Geometry: final body of the model. Coordinates: model frame, mm. Coordinates: 2 decimals unless noted, no trailing zeros. Loops run counter-clockwise (first coordinate to the right, second up) from the corner with the lowest first, then second, coordinate; pieces in that order, holes last. Notation, with made-up numbers: M 58,29 L 110,29 A28 ccw 110,68 Z; hole C 42,-34 d3. An arc over 180 degrees is marked long. Write each question's results on one line, items separated by ' | '. Start each with the question number.
from build123d import *
from build123d.topology import SkipClean

# Parameters (mm, degrees)
THICKEN1_START     = 3.38125
THICKEN1_DEPTH     = 22.11875
THICKEN1_2_DEPTH   = 1
THICKEN1_START_2   = 1.79375
THICKEN1_3_DEPTH   = 0.79375
THICKEN1_START_3   = 1
THICKEN1_4_DEPTH   = 2.38125
SKETCH7_R          = 0.396875
CUT_EXTRUDE1_DEPTH = 10


with BuildPart() as part:
    # Thicken1: read off the stored shape, not the designer's step
    # Thicken1 outline → Thicken1 (new body)
    with BuildSketch(Plane.XY.offset(THICKEN1_START)):
        with BuildLine():
            ThreePointArc((0, -0.794033341), (0.622, -0.172033341), (0, 0.449966659))
            Line((0, 0.449966659), (0, 0.348580659))
            ThreePointArc((0, 0.348580659), (0.520614, -0.172033341), (0, -0.692647341))
            Line((0, -0.692647341), (0, -0.794033341))
        make_face()
    extrude(amount=THICKEN1_DEPTH)



with BuildPart() as body_2:
    # Thicken1 2 outline → Thicken1 2 (new body)
    with BuildSketch(Plane.XY):
        with BuildLine():
            ThreePointArc((0, -0.794033341), (0.622, -0.172033341), (0, 0.449966659))
            Line((0, 0.449966659), (0, 0.348580659))
            ThreePointArc((0, 0.348580659), (0.520614, -0.172033341), (0, -0.692647341))
            Line((0, -0.692647341), (0, -0.794033341))
        make_face()
    extrude(amount=THICKEN1_2_DEPTH)


with BuildPart() as body_3:
    # Thicken1 3 outline → Thicken1 3 (new body)
    with BuildSketch(Plane.XY.offset(THICKEN1_START_2)):
        with BuildLine():
            ThreePointArc((0, -0.794033341), (0.622, -0.172033341), (0, 0.449966659))
            Line((0, 0.449966659), (0, 0.348580659))
            ThreePointArc((0, 0.348580659), (0.520614, -0.172033341), (0, -0.692647341))
            Line((0, -0.692647341), (0, -0.794033341))
        make_face()
    extrude(amount=THICKEN1_3_DEPTH)


with BuildPart() as part_1:
    add(part.part)

    add(body_2.part)  # Thicken1 4 merges body 2

    add(body_3.part)  # Thicken1 4 merges body 3
    # Thicken1 4 outline → Thicken1 4 (add)
    with BuildSketch(Plane.XY.offset(THICKEN1_START_3)):
        with BuildLine():
            Line((0.40339385, 0.157075059), (0.481952031, 0.221166659))
            ThreePointArc((0.481952031, 0.221166659), (0.26675232, 0.389862735), (0, 0.449966659))
            Line((0, 0.449966659), (0, 0.348580659))
            ThreePointArc((0, 0.348580659), (0.223271692, 0.298273674), (0.40339385, 0.157075059))
        make_face()
    extrude(amount=THICKEN1_4_DEPTH)

    # Sketch7 → Cut-Extrude1 (cut)
    with BuildSketch(Plane(origin=(0, 0, 0), x_dir=(1, 0, 0), z_dir=(0, 1, 0))):
        with Locations((0, -0.5)):
            Circle(SKETCH7_R)
    extrude(amount=-CUT_EXTRUDE1_DEPTH, mode=Mode.SUBTRACT)

    # Mirror2: part across face


with BuildPart() as part_2:
    with SkipClean():  # the faces are left unmerged after this step: merging them gives an invalid solid
        add(part_1.part)
        add(part_1.part.mirror(Plane(origin=(0, 0.399273659, 12.75), x_dir=(0, 0, 1), z_dir=(-1, 0, 0))))


solid = part_2.part
Item 1: Section A-A, the plane x = 0.2. Return loops of the section in (y, z).
Item 2: Section C-C, the plane z = 21. Return loops of the section in (x, y).
Item 3: Section D-D, the plane z = 0.5. Return loops of the section in (x, y), plus the area to 3 significant figures.
Item 4: Ray query, L1, parallel to Z at x = 0.5, y = 0.15; L2, parallel to Y at x = 0.45, z = 11.5. Return the intervals inside material, ascending. Write a range as [from, to].
Item 5: Section B-B, the plane y = -0.1. Return loops of the section in (x, z), plus the area to 3 significant figures.
Solutions:
1) outline: M -0.76,0 L -0.65,0 L -0.65,0.16 L -0.76,0.16 Z; M -0.76,0.84 L -0.65,0.84 L -0.65,1 L -0.76,1 Z; M -0.76,1.79 L -0.65,1.79 L -0.65,2.59 L -0.76,2.59 Z; M -0.76,3.38 L -0.65,3.38 L -0.65,25.5 L -0.76,25.5 Z; M 0.31,0 L 0.42,0 L 0.42,25.5 L 0.31,25.5 Z
2) outline: C 0,-0.17 d1.24; hole C 0,-0.17 d1.04
3) outline: M -0.4,-0.65 L -0.4,-0.51 A0.52 cw long 0.4,-0.51 L 0.4,-0.65 A0.62 ccw long Z | area: 0.275 mm²
4) L1: z = [0, 1], [1.79, 2.59], [3.38, 25.5] | L2: y = [-0.6, -0.43], [0.09, 0.26]
5) outline: M -0.62,0 L -0.52,0 L -0.52,1 L -0.62,1 Z; M -0.62,1.79 L -0.52,1.79 L -0.52,2.59 L -0.62,2.59 Z; M -0.62,3.38 L -0.52,3.38 L -0.52,25.5 L -0.62,25.5 Z; M 0.52,0 L 0.62,0 L 0.62,1 L 0.52,1 Z; M 0.52,1.79 L 0.62,1.79 L 0.62,2.59 L 0.52,2.59 Z; M 0.52,3.38 L 0.62,3.38 L 0.62,25.5 L 0.52,25.5 Z | area: 4.89 mm²
